```python
from build123d import *

# Parameters (mm, degrees)
ESQUISSE1_R                  = 40
BOSS_EXTRU_1_DEPTH           = 87
CONG_1_R                     = 40
ESQUISSE2_OUTSIDE_W          = 110.544
ESQUISSE2_OUTSIDE_H          = 110.544
ESQUISSE2_OUTSIDE_R          = 38
ENL_V_MAT_EXTRU_1_DEPTH      = 25
ENL_V_START                  = 40
ESQUISSE3_W                  = 76
ESQUISSE3_H                  = 19
ENL_V_MAT_EXTRU_2_DEPTH      = 10
ENL_V_MAT_EXTRU_3_DEPTH      = 20
ENL_V_MAT_EXTRU_4_DEPTH      = 68
ENL_V_MAT_EXTRU_5_REACH      = 21
ENL_V_MAT_EXTRU_5_END_RADIUS = 40
ESQUISSE6_R                  = 3.1
ESQUISSE8_R                  = 5.25
ENL_V_MAT_EXTRU_6_DEPTH      = 6
TROU_TARAUD_M2_51_D          = 2.05
TROU_TARAUD_M2_51_DEPTH      = 12
TROU_TARAUD_M51_REACH        = 25
TROU_TARAUD_M51_BORE_R       = 2.1


with BuildPart() as part:
    # Esquisse1 → Boss.-Extru.1 (new body)
    with BuildSketch(Plane(origin=(0, 0, 0), x_dir=(1, 0, 0), z_dir=(0, 1, 0))):
        with Locations(Location((0, 0, 0), (0, 0, 270))):  # turned: the seam where the file's is
            Circle(ESQUISSE1_R)
    extrude(amount=BOSS_EXTRU_1_DEPTH)

    # Congé1
    cong_1_edges = [part.edges().sort_by_distance(p)[0] for p in [
        (0, 87, -40),
    ]]
    fillet(cong_1_edges, radius=CONG_1_R)

    # Esquisse2 outside → Enlèv. mat.-Extru.1 (cut)
    with BuildSketch(Plane.XZ):
        Rectangle(ESQUISSE2_OUTSIDE_W, ESQUISSE2_OUTSIDE_H)
        with Locations(Location((0, 0, 0), (0, 0, 270))):  # turned: the seam where the file's is
            Circle(ESQUISSE2_OUTSIDE_R, mode=Mode.SUBTRACT)
    extrude(amount=-ENL_V_MAT_EXTRU_1_DEPTH, mode=Mode.SUBTRACT)

    # Esquisse3 → Enlèv. mat.-Extru.2 (cut)
    with BuildSketch(Plane.XY.offset(ENL_V_START)):
        with Locations((0, 42.5)):
            Rectangle(ESQUISSE3_W, ESQUISSE3_H)
    extrude(amount=-ENL_V_MAT_EXTRU_2_DEPTH, mode=Mode.SUBTRACT)

    # Esquisse4 → Enlèv. mat.-Extru.3 (cut)
    with BuildSketch(Plane.XY.offset(30)):
        with BuildLine():
            Line((-6.5, 36.5), (6.5, 36.5))
            ThreePointArc((6.5, 36.5), (9.328427125, 37.671572875), (10.5, 40.5))
            Line((10.5, 40.5), (10.5, 44.5))
            ThreePointArc((10.5, 44.5), (9.328427125, 47.328427125), (6.5, 48.5))
            Line((6.5, 48.5), (-6.5, 48.5))
            ThreePointArc((-6.5, 48.5), (-9.328427125, 47.328427125), (-10.5, 44.5))
            Line((-10.5, 44.5), (-10.5, 40.5))
            ThreePointArc((-10.5, 40.5), (-9.328427125, 37.671572875), (-6.5, 36.5))
        make_face()
    extrude(amount=-ENL_V_MAT_EXTRU_3_DEPTH, mode=Mode.SUBTRACT)

    # Esquisse5 → Enlèv. mat.-Extru.4 (cut)
    with BuildSketch(Plane.XZ):
        Polygon((-14, 18), (16, 18), (16, 22), (24, 22), (24, -22), (16, -22), (16, -18), (-14, -18), (-14, -20.5), (-17, -20.5), (-17, -18), (-27, -8), (-27, 8), (-17, 18), (-17, 20.5), (-14, 20.5), align=None)
    extrude(amount=-ENL_V_MAT_EXTRU_4_DEPTH, mode=Mode.SUBTRACT)

    # Enlèv. mat.-Extru.5: up to this sphere (the profile starts inside it)
    enl_v_mat_extru_5_end = Location((0, 47, 0)) * Sphere(ENL_V_MAT_EXTRU_5_END_RADIUS, mode=Mode.PRIVATE)
    # Esquisse6 → Enlèv. mat.-Extru.5 (cut, up to the surface)
    with BuildSketch(Plane.XZ.offset(-68), mode=Mode.PRIVATE) as enl_v_mat_extru_5_sk1:
        with Locations(Location((0, 0, 0), (0, 0, 270))):  # turned: the seam where the file's is
            Circle(ESQUISSE6_R)
    enl_v_mat_extru_5_tool1 = extrude(enl_v_mat_extru_5_sk1.sketch, amount=-ENL_V_MAT_EXTRU_5_REACH, mode=Mode.PRIVATE) & enl_v_mat_extru_5_end
    add(enl_v_mat_extru_5_tool1.solids().sort_by_distance((0, 68, 0))[0], mode=Mode.SUBTRACT)

    # Esquisse8 → Enlèv. mat.-Extru.6 (cut)
    with BuildSketch(Plane.XZ.offset(-87)):
        with Locations(Location((0, 0, 0), (0, 0, 270))):  # turned: the seam where the file's is
            Circle(ESQUISSE8_R)
    extrude(amount=ENL_V_MAT_EXTRU_6_DEPTH, mode=Mode.SUBTRACT)

    # Esquisse11 → Enlèvement de matière-Révolution1 (revolve, cut)
    with BuildSketch(Plane.XY, mode=Mode.PRIVATE) as enl_vement_de_mati_re_r_volution1_sk:
        Polygon((-27, 47), (-27, 41), (-45, 30.607695155), (-45, 47), align=None)
    revolve(enl_vement_de_mati_re_r_volution1_sk.sketch.rotate(Axis((-27, 47, 0), (-1, 0, 0)), 270), axis=Axis((-27, 47, 0), (-1, 0, 0)), mode=Mode.SUBTRACT)  # turned: the seam where the file's is

    # Trou taraudé M2.51
    with Locations(Plane.XY.offset(30)):
        with Locations((-12.5, 42.5), (12.5, 42.5)):
            Hole(TROU_TARAUD_M2_51_D / 2, depth=TROU_TARAUD_M2_51_DEPTH)

    # Trou taraudé M51 bore → Trou taraudé M51 (cut, up to next)
    with BuildSketch(Plane(origin=(-17, 0, 0), x_dir=(0, 0, -1), z_dir=(1, 0, 0)), mode=Mode.PRIVATE) as trou_taraud_m51_sk1:
        with Locations((14, 21)):
            Circle(TROU_TARAUD_M51_BORE_R)
    trou_taraud_m51_tool1 = extrude(trou_taraud_m51_sk1.sketch, amount=-TROU_TARAUD_M51_REACH, mode=Mode.PRIVATE) & part.part
    add(trou_taraud_m51_tool1.solids().sort_by_distance((-17, 21, -14))[0], mode=Mode.SUBTRACT)


solid = part.part
```
For this review, take the finished solid that the model builds, in its own axes (mm). A direction names the side the tool comes from. Coordinates: 2 decimals unless noted, no trailing zeros. Write each loop counter-clockwise with the first axis right and the second up, starting at its lowest first coordinate (ties: lowest second). Pieces come first, ordered by that corner, then holes. Notation, with made-up numbers: (69, 67.5) - (94, 67.5) arc R18 cw to (94, 77.5) - close; hole circle Ø9 at (44, 60.5). An arc over 180 degrees is marked (long way). Answer in a Markdown table with one row per item. Add a question column.
Q1. We need section C-C, the plane y = 17. State the section outline as (x, z) points, and give its area (3 significant figures).
Q2. Draft analysis for pull direction Z (two halves, no side actions). For faces 1 (the flat face through (20, 34, -22)), 2 (the flat face through (0, 36, 30)), 3 (the cylindrical face through (9.359, 47.297, 24.084)), state which applies: +Z half, -Z half, draft (parallel to the pull), parting line (faces both ways), or undercut.
Q3. For probe 1 along X at (y, z) = (22, -0.5); probe 2 along Z at (x, y) = (-25, 21); probe 3 along X at (y, z) = (42, 21), list the stretches that pass through material, from the lowest coordinate up.
Q4. We need section B-B, the plane x = 0. State the section outline as (y, z) points.
Q5. We need section D-D, the plane x = -24. State the section outline as (y, z) points, and give its area (3 significant figures).
Q6. We need section A-A, the plane z = 0. State the section outline as (x, y) points, and give its area (3 significant figures).
Q7. Tool access review of faces 4 (the cylindrical face through (1.6, 83.9, -5)), 5 (the flat face through (0, 33, 34)), 6 (the cylindrical face through (-27.374, 21.631, -16.003)), 7 (the flat face through (-22, 34, 13)), 8 (the cylindrical face through (-9.297, 47.359, 24.084)): name each direction out of +Z, -Z, +X, -X, +Y, -Y from which nothing blocks a thin tool from reaching the whole face with its end or side.
Q8. For P1, Ø4, axis at y = 45, z = -24, coming from the -X side; P2, Ø10, axis at x = 26.5, z = 14.5, coming from the +Y side; P3, Ø12, axis at y = 9, z = -13.5, coming from the +X side; P4, Ø9, axis at x = 0.5, y = 33.5, coming from the -Z side, all flat-tipped, find the tip position at first contact; note any pin that passes through.
Answer list:
| question | item | result |
|---|---|---|
| 1 | outline | circle Ø76 at (0, 0); hole (-27, -8) - (-17, -18) - (-17, -20.5) - (-14, -20.5) - (-14, -18) - (16, -18) - (16, -22) - (24, -22) - (24, 22) - (16, 22) - (16, 18) - (-14, 18) - (-14, 20.5) - (-17, 20.5) - (-17, 18) - (-27, 8) - close |
| 1 | area | 2,720 mm2 |
| 2 | face 1 | undercut |
| 2 | face 2 | +Z half |
| 2 | face 3 | draft |
| 3 | probe 1 | x = -38 to -27, 24 to 38 |
| 3 | probe 2 | z = -28.62 to -16.1, -11.9 to -10, 10 to 28.62 |
| 3 | probe 3 | x = -34.04 to -13.39, -11.61 to -10.5, 10.5 to 11.61, 13.39 to 16, 24 to 34.04 |
| 4 | outline | (0, -38) - (25, -38) - (25, -40) - (47, -40) arc R40 ccw to (86.65, -5.25) - (81, -5.25) - (81, -3.1) - (68, -3.1) - (68, -18) - (0, -18) - close; (0, 18) - (36.5, 18) - (36.5, 30) - (33, 30) - (33, 40) - (25, 40) - (25, 38) - (0, 38) - close; (48.5, 18) - (68, 18) - (68, 3.1) - (81, 3.1) - (81, 5.25) - (86.65, 5.25) arc R40 ccw to (52, 39.69) - (52, 30) - (48.5, 30) - close |
| 5 | outline | (0, -29.46) - (25, -29.46) - (25, -32) - (47, -32) arc R32 ccw to (52, 31.61) - (52, 30) - (33, 30) - (33, 32) - (25, 32) - (25, 29.46) - (0, 29.46) - (0, 11) - (68, 11) - (68, -11) - (0, -11) - close; hole circle Ø4.2 at (21, -14) |
| 5 | area | 2,940 mm2 |
| 6 | outline | (-40, 25) - (-38, 25) - (-38, 0) - (-27, 0) - (-27, 41) - (-40, 33.49) - close; (-38.04, 59.37) - (-27, 53) - (-27, 68) - (-3.1, 68) - (-3.1, 81) - (-5.25, 81) - (-5.25, 86.65) arc R40 ccw to start; (3.1, 68) - (24, 68) - (24, 0) - (38, 0) - (38, 25) - (40, 25) - (40, 47) arc R40 ccw to (5.25, 86.65) - (5.25, 81) - (3.1, 81) - close |
| 6 | area | 2,320 mm2 |
| 7 | face 4 | +Y |
| 7 | face 5 | +Z, +X, -X |
| 7 | face 6 | -X |
| 7 | face 7 | -Y |
| 7 | face 8 | +Z |
| 8 | P1 | stops at x = -33.41 |
| 8 | P2 | stops at y = 78.06 |
| 8 | P3 | stops at x = 37.25 |
| 8 | P4 | stops at z = -40 |
